Input: part model. Units: mm. Frame: model coordinates. Face numbers are marked on the shaded views. A direction names the side the tool comes from. Coordinates: 2 decimals unless noted, no trailing zeros. Order: outer loops, then holes, each group sorted by start corner. A loop starts at its lowest first (then second) coordinate and runs counter-clockwise, first axis right, second up.
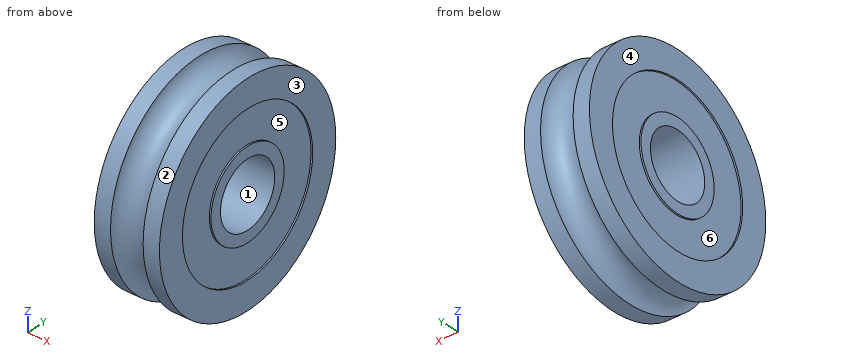
from build123d import *

# Parameters (mm, degrees)
SKETCH2_R          = 2
CUT_EXTRUDE1_DEPTH = 11.024968828
SKETCH3_R          = 4.8
SKETCH3_R_2        = 2.7
CUT_EXTRUDE2_DEPTH = 0.1


with BuildPart() as part:
    # Sketch1 → Revolve1 (revolve)
    with BuildSketch(Plane.XY, mode=Mode.PRIVATE) as revolve1_sk:
        with BuildLine():
            Line((1, 6.5), (2, 6.5))
            Line((2, 6.5), (2, 0))
            Line((2, 0), (-2, 0))
            Line((-2, 0), (-2, 6.5))
            Line((-2, 6.5), (-1, 6.5))
            ThreePointArc((-1, 6.5), (0, 5.5), (1, 6.5))
        make_face()
    revolve(revolve1_sk.sketch.rotate(Axis((2, 0, 0), (1, 0, 0)), 180), axis=Axis((2, 0, 0), (1, 0, 0)))

    # Sketch2 → Cut-Extrude1 (cut, through all)
    with BuildSketch(Plane(origin=(2, 0, 0), x_dir=(0, 0, -1), z_dir=(1, 0, 0))):
        with Locations(Location((0, 0, 0), (0, 0, 90))):
            Circle(SKETCH2_R)
    extrude(amount=-CUT_EXTRUDE1_DEPTH, mode=Mode.SUBTRACT)

    # Sketch3 → Cut-Extrude2 (cut)
    with BuildSketch(Plane(origin=(2, 0, 0), x_dir=(0, 0, -1), z_dir=(1, 0, 0))):
        with Locations(Location((0, 0, 0), (0, 0, 90))):
            Circle(SKETCH3_R)
        with Locations(Location((0, 0, 0), (0, 0, 90))):
            Circle(SKETCH3_R_2, mode=Mode.SUBTRACT)
    cut_extrude2 = extrude(amount=-CUT_EXTRUDE2_DEPTH, mode=Mode.SUBTRACT)

    # Mirror1: Cut-Extrude2 across plane
    add(cut_extrude2.mirror(Plane(origin=(0, 0, 0), x_dir=(0, 0, 1), z_dir=(1, 0, 0))), mode=Mode.SUBTRACT)


solid = part.part
Item 1: Cut plane D-D on x = -0.05. Return loops of the section in (y, z), then the cut area to 3 significant figures.
Response values:
outline: circle Ø11 at (0, 0); hole circle Ø4 at (0, 0)
area: 82.5 mm2
Item 2: Access query for the marked faces 4, 5 and 6. Directions: +Z, -Z, +X, -X, +Y, -Y. A direction counts if a zero-diameter tool reaches every point of the face in a straight line with its end or side. Return the directions, or none.
Response values:
face 4: +Z, -Z, -X, +Y, -Y
face 5: +X
face 6: -X
Item 3: Cut plane C-C on x = 1.5. Return loops of the section in (y, z), then the cut area to 3 significant figures.
Response values:
outline: circle Ø13 at (0, 0); hole circle Ø4 at (0, 0)
area: 120 mm2
Item 4: Draft query along Z for the marked faces 1, 2 and 3. Return one class per face: pulls with the +Z half, pulls with the -Z half, needs draft (parallel to the pull), parting line crosses it, or undercut.
Response values:
face 1: undercut
face 2: parting line crosses it
face 3: needs draft
Item 5: Cut plane A-A on z = 0. Return loops of the section in (x, y).
Response values:
outline: (-2, -6.5) - (-1, -6.5) arc R1 cw to (1, -6.5) - (2, -6.5) - (2, -4.8) - (1.9, -4.8) - (1.9, -2.7) - (2, -2.7) - (2, -2) - (-2, -2) - (-2, -2.7) - (-1.9, -2.7) - (-1.9, -4.8) - (-2, -4.8) - close; (-2, 2) - (2, 2) - (2, 2.7) - (1.9, 2.7) - (1.9, 4.8) - (2, 4.8) - (2, 6.5) - (1, 6.5) arc R1 cw to (-1, 6.5) - (-2, 6.5) - (-2, 4.8) - (-1.9, 4.8) - (-1.9, 2.7) - (-2, 2.7) - close
Item 6: Ray query, probe 1 along Z at (x, y) = (-1.85, 0); probe 2 along X at (y, z) = (-1.25, 5.5); probe 3 along Z at (x, y) = (-1.7, -1.5). Return the intervals inside material, ascending.
Response values:
probe 1: z = -6.5 to -2, 2 to 6.5
probe 2: x = -2 to -0.51, 0.51 to 2
probe 3: z = -6.32 to -1.32, 1.32 to 6.32
Item 7: Pin query (flat end, axial travel): pin 1 Ø1 at (x, y) = (-1, 1) entering from -Z; pin 2 Ø3.5 at (y, z) = (0, 0) entering from +X. Return the tip coordinate at first contact, or that it passes through.
Response values:
pin 1: stops at z = -6.48
pin 2: passes through
